Here's how the part is built. I have some questions about the finished solid (model axes, mm). A direction names the side the tool comes from. Round coordinates to 2 decimals unless told otherwise and drop trailing zeros. Order: outer loops, then holes, each group sorted by start corner. A loop starts at its lowest first (then second) coordinate and runs counter-clockwise, first axis right, second up. Notation, with made-up numbers: (-22, 36.5) -> (-9, 36.5) arc R12 ccw to (-9, 59.5) -> close; hole circle Ø7 at (41.5, 16.25). An arc over 180 degrees is marked (long way). One line per item, written item: value.
```python
from build123d import *

# Parameters (mm, degrees)
F1_DEPTH = 4
F2_R     = 4
F2_R_2   = 1.45
F3_DEPTH = 4
F2_W     = 5
F2_H     = 64.0853656404
F2_H_2   = 12.9573171798
F4_DEPTH = 16
F5_R     = 2.25
F6_DEPTH = 25
F7_DEPTH = 4
F8_DEPTH = 25


with BuildPart() as f1:
    # F0 (on Top) → F1 (new body)
    with BuildSketch(Plane.XY):
        Polygon((32.6684095042, 32.6008076754), (-70.8834637033, 32.6008076754), (-70.8834637033, -31.4845579651), (-48.0820438839, -31.4845579651), (-48.0820438839, 16.5019411054), (32.6684095042, 16.5019411054), align=None)
    extrude(amount=-F1_DEPTH)

    # F2 (on face) → F3 (join)
    with BuildSketch(Plane(origin=(0, 0, -4), x_dir=(1, 0, 0), z_dir=(0, 0, -1))):
        with Locations((-53.3834637033, 25.3991923246)):
            Circle(F2_R)
        with Locations((-53.3834637033, 25.3991923246)):
            Circle(F2_R_2, mode=Mode.SUBTRACT)
        with Locations((26.6165362967, -22.6008076754)):
            Circle(F2_R)
        with Locations((26.6165362967, -22.6008076754)):
            Circle(F2_R_2, mode=Mode.SUBTRACT)
        with Locations((-53.3834637033, -22.6008076754)):
            Circle(F2_R)
    extrude(amount=F3_DEPTH)

    # F2 (on face) → F4 (join)
    with BuildSketch(Plane(origin=(0, 0, -4), x_dir=(1, 0, 0), z_dir=(0, 0, -1))):
        with Locations((-68.3834637033, -0.5581248552)):
            Rectangle(F2_W, F2_H)
        with Locations((-68.3834637033, 37.963216555)):
            Rectangle(F2_W, F2_H_2)
        with Locations((-68.3834637033, -39.0794662653)):
            Rectangle(F2_W, F2_H_2)
    extrude(amount=F4_DEPTH)

    # F5 (on face) → F6 (cut)
    with BuildSketch(Plane(origin=(-70.8834637033, 0, 0), x_dir=(0, -1, 0), z_dir=(-1, 0, 0))):
        with Locations((-36.1952548007, -10)):
            Circle(F5_R)
        with Locations((34.5479122297, -10)):
            Circle(F5_R)
    extrude(amount=-F6_DEPTH, mode=Mode.SUBTRACT)

    # F2 (on face) → F7 (join)
    with BuildSketch(Plane(origin=(0, 0, -4), x_dir=(1, 0, 0), z_dir=(0, 0, -1))):
        with Locations((-68.3834637033, 37.963216555)):
            Rectangle(F2_W, F2_H_2)
        with Locations((-68.3834637033, -39.0794662653)):
            Rectangle(F2_W, F2_H_2)
    extrude(amount=-F7_DEPTH)

    # F2 (on face) → F8 (cut)
    with BuildSketch(Plane(origin=(0, 0, -4), x_dir=(1, 0, 0), z_dir=(0, 0, -1))):
        with Locations((-53.3834637033, 25.3991923246)):
            Circle(F2_R_2)
        with Locations((26.6165362967, -22.6008076754)):
            Circle(F2_R_2)
    extrude(amount=-F8_DEPTH, mode=Mode.SUBTRACT)


solid = f1.part
```
Q1. I need wall thicknesses on line 1 along X through (y, z) = (28, -18.5); line 2 along Z through (x, y) = (-45.5, 27); line 3 along X through (y, z) = (-3, -3.25). Which ranges of each line are inside material? Lowest first, please.
Answers:
line 1: -70.88 to -65.88
line 2: -4 to 0
line 3: -70.88 to -48.08
Q2. For P1, Ø2.5, axis at y = -34.55, z = -10, coming from the -X side; P2, Ø4, axis at x = -54, y = 22.5, coming from the -Z side; P3, Ø1, axis at x = -2, y = 30.5, coming from the -Z side; P4, Ø3, axis at x = 7.5, z = -1.5, coming from the +Y side, each with a flat end and sliding along its axis, tell me the tip position at first contact or that it passes through.
Answers:
P1: through
P2: z = -8
P3: z = -4
P4: y = 32.6
Q3. I want a section at A-A on z = -10. Write out the boundary of the cut face in (x, y).
Answers:
outline: (-70.88, -44.44) -> (-65.88, -44.44) -> (-65.88, -36.8) -> (-70.88, -36.8) -> close; (-70.88, -32.3) -> (-65.88, -32.3) -> (-65.88, 33.95) -> (-70.88, 33.95) -> close; (-70.88, 38.45) -> (-65.88, 38.45) -> (-65.88, 45.56) -> (-70.88, 45.56) -> close
Q4. I want a section at D-D on z = -16. Write out the boundary of the cut face in (x, y), then the cut area to 3 significant figures.
Answers:
outline: (-70.88, -44.44) -> (-65.88, -44.44) -> (-65.88, 45.56) -> (-70.88, 45.56) -> close
area: 450 mm2
Q5. Which directions (+Z, -Z, +X, -X, +Y, -Y) give clear straight access to the entire face, cutting with the end or side of a thin tool? Please do faces 1 (the face through (28.77, 19.23, -5.97)), 2 (the face through (-8, 16.502, -2)), 3 (the face through (-51.7, -25.5, -8)), 4 (the face through (32.668, 24, -2)).
Answers:
face 1: -Z
face 2: +Z, -Z, +X, -Y
face 3: -Z, +X, +Y, -Y
face 4: +Z, -Z, +X, +Y, -Y
Q6. If we mould it in two halves opening along Y, with no side actions, what happens to faces 5 (the face through (-68.42, 34.99, -8.1)), 6 (the face through (26.6, 24.3, -8)), 7 (the face through (-16, 32.601, -2)), 8 (the face through (-68.4, -32.3, -9.9))? For each: pulls with the +Y half, pulls with the -Y half, needs draft (parallel to the pull), parting line crosses it, or undercut.
Answers:
face 5: undercut
face 6: needs draft
face 7: pulls with the +Y half
face 8: undercut
Q7. I want a section at B-B on y = -1.5. Write out the boundary of the cut face in (x, z), then the cut area to 3 significant figures.
Answers:
outline: (-70.88, -20) -> (-65.88, -20) -> (-65.88, -4) -> (-48.08, -4) -> (-48.08, 0) -> (-70.88, 0) -> close
area: 171 mm2
Q8. I want a section at C-C on x = -1.5. Write out the boundary of the cut face in (y, z).
Answers:
outline: (16.5, -4) -> (32.6, -4) -> (32.6, 0) -> (16.5, 0) -> close
